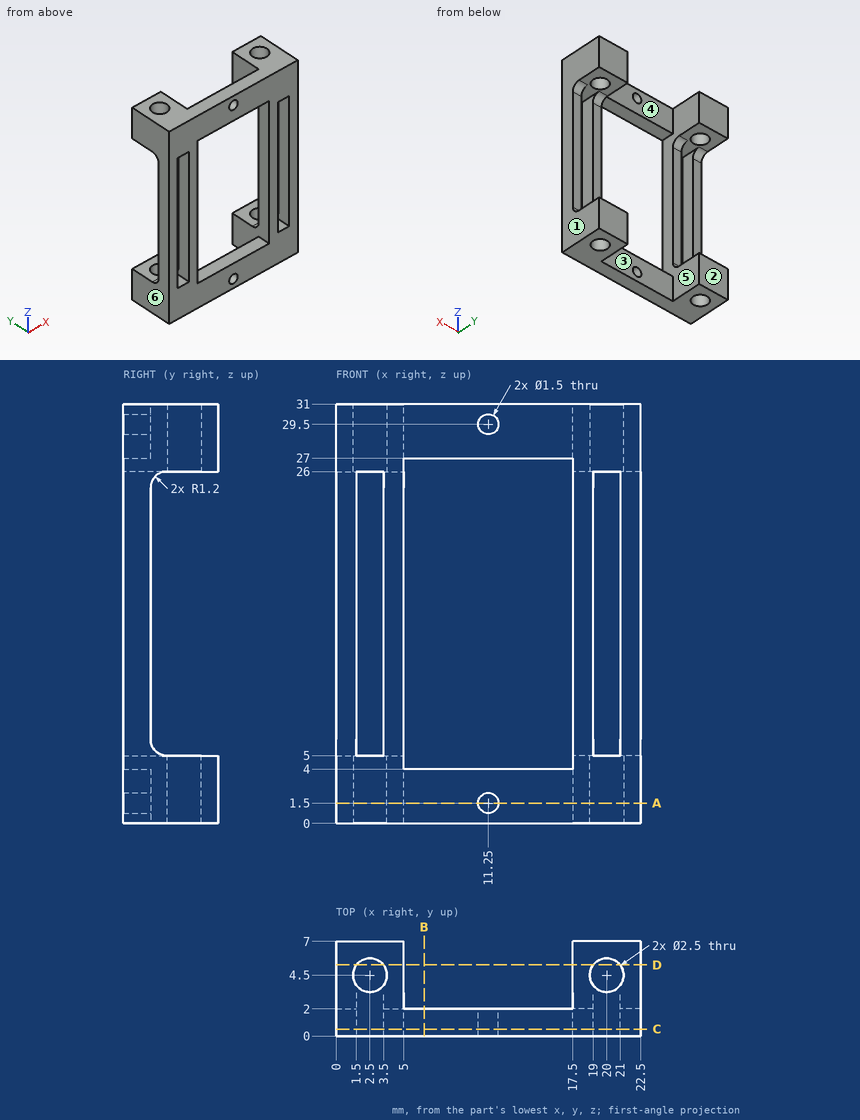
Part print with two shaded views. Sizes in mm from the minimum x, y, z corner. A direction names the side the tool comes from. Coordinates: 2 decimals unless noted, no trailing zeros. Write each loop counter-clockwise with the first axis right and the second up, starting at its lowest first coordinate (ties: lowest second). Pieces come first, ordered by that corner, then holes.
(1) Cut at B-B on x = 6.5. List the corners of the cut face in (y, z), and give its area (3 significant figures).
(2) Cut at D-D on y = 5.25. State how many separate pieces and enclosed holes the cut face has, and give its area (3 significant figures).
(3) Cut at C-C on y = 0.5. List the corners of the cut face in (x, z), and give its area (3 significant figures).
(4) Drill centre lines: line 1 (X direction, y = 1.5, z = 15.5); line 2 (Z direction, x = 11.25, y = 1); line 3 (X direction, y = 3, z = 27.5). Where is each one in solid material? Low to high.
(5) Cut at A-A on z = 1.5. List the corners of the cut face in (x, y).
(6) Pin check, flat tips, straight feed: pin 1 Ø1.5 at (x, y) = (20, 2.5) entering from -Z; pin 2 Ø1.2 at (x, z) = (18, 18.5) entering from +Y; pin 3 Ø1.5 at (y, z) = (3.5, 9) entering from -X. Stop position of each tip, or through.
(7) Mould opens along X. For the marked faces 1, 2 and 3 say: pulls with the +X half, pulls with the -X half, needs draft (parallel to the pull), parting line crosses it, or undercut.
(8) 3-axis set-ups, long thin cutter, end or side, ignore diameter. For the marked faces 4, 5 and 6: which of +Z, -Z, +X, -X, +Y, -Y reach the whole face in a straight line?
Working result:
1. outline: (0, 0) - (2, 0) - (2, 4) - (0, 4) - close; (0, 27) - (2, 27) - (2, 31) - (0, 31) - close
1. area: 16.0 mm2
2. separate pieces: 8
2. enclosed holes: 0
2. area: 60.0 mm2
3. outline: (0, 0) - (22.5, 0) - (22.5, 31) - (0, 31) - close; hole (1.5, 5) - (3.5, 5) - (3.5, 26) - (1.5, 26) - close; hole (5, 4) - (17.5, 4) - (17.5, 27) - (5, 27) - close; hole circle Ø1.5 at (11.25, 1.5); hole circle Ø1.5 at (11.25, 29.5); hole (19, 5) - (21, 5) - (21, 26) - (19, 26) - close
3. area: 322 mm2
4. line 1: x = 0 to 1.5, 3.5 to 5, 17.5 to 19, 21 to 22.5
4. line 2: z = 0 to 0.75, 2.25 to 4, 27 to 28.75, 30.25 to 31
4. line 3: x = 0 to 5, 17.5 to 22.5
5. outline: (0, 0) - (10.5, 0) - (10.5, 2) - (5, 2) - (5, 7) - (0, 7) - close; (12, 0) - (22.5, 0) - (22.5, 7) - (17.5, 7) - (17.5, 2) - (12, 2) - close; hole circle Ø2.5 at (2.5, 4.5); hole circle Ø2.5 at (20, 4.5)
6. pin 1: stops at z = 0
6. pin 2: stops at y = 2
6. pin 3: passes through
7. face 1: pulls with the +X half
7. face 2: needs draft
7. face 3: undercut
8. face 4: +Z, -Z, +Y
8. face 5: +Y
8. face 6: +Z, -Z, -X, +Y, -Y
